CAD build for the part. Positions are in the model's coordinates, mm. Face numbers are marked on the shaded views. A direction names the side the tool comes from. Round coordinates to 2 decimals unless told otherwise and drop trailing zeros. Write each loop counter-clockwise with the first axis right and the second up, starting at its lowest first coordinate (ties: lowest second). Pieces come first, ordered by that corner, then holes. Notation, with made-up numbers: (34.5, -37) - (78.5, -37) arc R17 ccw to (78.5, -4) - close; hole circle Ø5 at (-20.5, -11.75). An arc over 180 degrees is marked (long way). Use one line per item in the form item = value. Start each with the question number.
Item 1: Drill centre lines: L1, parallel to X at y = 18, z = -43.5; L2, parallel to X at y = 23, z = -108; L3, parallel to Z at x = -30.5, y = 20. Where is each one in solid material? Low to high.
Item 2: Band-saw the part on B-B, the plane z = -60. Give the number of separate pieces and of enclosed holes in the cut face, and give its area (4 significant figures).
Item 3: Pull direction X, two halves, no side cores. Call the marked faces 3, 4 and 5: +X half, -X half, draft (parallel to the pull), parting line (faces both ways), or undercut.
Item 4: Pin check, flat tip, straight feed: pin 1 (12 mm diameter, centred on x = 1.5, z = 49, fed in from +Y). Stop position of the tip, or through.
Item 5: Band-saw the part on A-A, the plane x = -16.5. List the corners of the cut face in (y, z).
Item 6: Tool access for the marked faces 1 and 2: list every direction of +Z, -Z, +X, -X, +Y, -Y with a clear straight run to the whole face (end or side of a thin tool).
from build123d import *

# Parameters (mm, degrees)
BOSS_EXTRUDE1_DEPTH     = 6.35
BOSS_EXTRUDE2_DEPTH     = 38.1
CUT_EXTRUDE1_DEPTH      = 12.7
CUT_EXTRUDE1_DEPTH_BACK = 25.4
CUT_EXTRUDE2_DEPTH      = 6.35
CUT_EXTRUDE2_DEPTH_BACK = 25.4
CUT_EXTRUDE3_DEPTH      = 156.552724943
BOSS_EXTRUDE3_DEPTH     = 38.1


with BuildPart() as part:
    # Sketch1 → Boss-Extrude1 (new body)
    with BuildSketch(Plane(origin=(0, 0, 0), x_dir=(1, 0, 0), z_dir=(0, 1, 0))):
        with BuildLine():
            Line((-81.75625, 119.0625), (81.75625, 119.0625))
            ThreePointArc((81.75625, 119.0625), (87.368910076, 116.737660076), (89.69375, 111.125))
            Line((89.69375, 111.125), (89.69375, -93.6625))
            ThreePointArc((89.69375, -93.6625), (82.254262242, -111.623012242), (64.29375, -119.0625))
            Line((64.29375, -119.0625), (-64.29375, -119.0625))
            ThreePointArc((-64.29375, -119.0625), (-82.254262242, -111.623012242), (-89.69375, -93.6625))
            Line((-89.69375, -93.6625), (-89.69375, 111.125))
            ThreePointArc((-89.69375, 111.125), (-87.368910076, 116.737660076), (-81.75625, 119.0625))
        make_face()
    extrude(amount=BOSS_EXTRUDE1_DEPTH)

    # Sketch2 → Boss-Extrude2 (add)
    with BuildSketch(Plane(origin=(0, 6.35, 0), x_dir=(1, 0, 0), z_dir=(0, 1, 0))):
        with BuildLine():
            Line((89.69375, -93.6625), (89.69375, 111.125))
            ThreePointArc((89.69375, 111.125), (87.368910076, 116.737660076), (81.75625, 119.0625))
            Line((81.75625, 119.0625), (-81.75625, 119.0625))
            ThreePointArc((-81.75625, 119.0625), (-87.368910076, 116.737660076), (-89.69375, 111.125))
            Line((-89.69375, 111.125), (-89.69375, -93.6625))
            ThreePointArc((-89.69375, -93.6625), (-82.254262242, -111.623012242), (-64.29375, -119.0625))
            Line((-64.29375, -119.0625), (64.29375, -119.0625))
            ThreePointArc((64.29375, -119.0625), (82.254262242, -111.623012242), (89.69375, -93.6625))
        make_face()
        with BuildLine():
            Line((81.75625, 112.7125), (-81.75625, 112.7125))
            ThreePointArc((-81.75625, 112.7125), (-82.878782015, 112.247532015), (-83.34375, 111.125))
            Line((-83.34375, 111.125), (-83.34375, -93.6625))
            ThreePointArc((-83.34375, -93.6625), (-77.764134182, -107.132884182), (-64.29375, -112.7125))
            Line((-64.29375, -112.7125), (64.29375, -112.7125))
            ThreePointArc((64.29375, -112.7125), (77.764134182, -107.132884182), (83.34375, -93.6625))
            Line((83.34375, -93.6625), (83.34375, 111.125))
            ThreePointArc((83.34375, 111.125), (82.878782015, 112.247532015), (81.75625, 112.7125))
        make_face(mode=Mode.SUBTRACT)
    extrude(amount=BOSS_EXTRUDE2_DEPTH)

    # Sketch5 → Cut-Extrude1 (cut, two sides: drawn at the far end of the back side and taken through both)
    with BuildSketch(Plane(origin=(-13.135345572, 31.711529428, 0), x_dir=(0, 0, 1), z_dir=(-0.38268343236509383, 0.9238795325112852, 0)).offset(-CUT_EXTRUDE1_DEPTH_BACK)):
        with BuildLine():
            Line((-52.21366875, -70.394979916), (-11.28633125, -70.394979916))
            add(Edge.make_bspline(
                [(-11.28633125, -70.394979916), (20.46366875, -70.394979916), (20.46366875, -38.644979916), (-11.28633125, -38.644979916)],
                knots=[0, 0, 0, 0, 1, 1, 1, 1], degree=3, weights=[1, 0.333333333, 0.333333333, 1]))
            Line((-11.28633125, -38.644979916), (-52.21366875, -38.644979916))
            add(Edge.make_bspline(
                [(-52.21366875, -70.394979916), (-83.96366875, -70.394979916), (-83.96366875, -38.644979916), (-52.21366875, -38.644979916)],
                knots=[0, 0, 0, 0, 1, 1, 1, 1], degree=3, weights=[1, 0.333333333, 0.333333333, 1]))
        make_face()
    extrude(amount=CUT_EXTRUDE1_DEPTH + CUT_EXTRUDE1_DEPTH_BACK, mode=Mode.SUBTRACT)

    # Sketch7 → Cut-Extrude2 (cut, two sides: drawn at the far end of the back side and taken through both)
    with BuildSketch(Plane(origin=(13.135345572, 31.711529428, 0), x_dir=(0, 0, -1), z_dir=(0.3826834323650874, 0.9238795325112878, 0)).offset(-CUT_EXTRUDE2_DEPTH_BACK)):
        with BuildLine():
            Line((10.20445, -72.146741698), (53.29555, -72.146741698))
            add(Edge.make_bspline(
                [(53.29555, -40.396741698), (85.04555, -40.396741698), (85.04555, -72.146741698), (53.29555, -72.146741698)],
                knots=[0, 0, 0, 0, 1, 1, 1, 1], degree=3, weights=[1, 0.333333333, 0.333333333, 1]))
            Line((53.29555, -40.396741698), (10.20445, -40.396741698))
            add(Edge.make_bspline(
                [(10.20445, -72.146741698), (-21.54555, -72.146741698), (-21.54555, -40.396741698), (10.20445, -40.396741698)],
                knots=[0, 0, 0, 0, 1, 1, 1, 1], degree=3, weights=[1, 0.333333333, 0.333333333, 1]))
        make_face()
    extrude(amount=CUT_EXTRUDE2_DEPTH + CUT_EXTRUDE2_DEPTH_BACK, mode=Mode.SUBTRACT)

    # Sketch8 → Cut-Extrude3 (cut, through all)
    with BuildSketch(Plane.XZ):
        with BuildLine():
            Line((13.49375, 106.83875), (26.19375, 106.83875))
            ThreePointArc((26.19375, 106.83875), (35.71875, 97.31375), (26.19375, 87.78875))
            Line((26.19375, 87.78875), (13.49375, 87.78875))
            ThreePointArc((13.49375, 87.78875), (3.96875, 97.31375), (13.49375, 106.83875))
        make_face()
        with BuildLine():
            Line((-26.19375, 80.9625), (-13.49375, 80.9625))
            ThreePointArc((-13.49375, 80.9625), (-3.96875, 71.4375), (-13.49375, 61.9125))
            Line((-13.49375, 61.9125), (-26.19375, 61.9125))
            ThreePointArc((-26.19375, 61.9125), (-35.71875, 71.4375), (-26.19375, 80.9625))
        make_face()
    extrude(amount=-CUT_EXTRUDE3_DEPTH, mode=Mode.SUBTRACT)

    # Sketch9 → Boss-Extrude3 (add)
    with BuildSketch(Plane(origin=(0, 6.35, 0), x_dir=(1, 0, 0), z_dir=(0, 1, 0))):
        with BuildLine():
            Line((-81.75625, 112.7125), (-71.120073585, 112.7125))
            ThreePointArc((-71.120073585, 112.7125), (-73.309655038, 111.836708137), (-74.291288385, 109.692489328))
            ThreePointArc((-74.291288385, 109.692489328), (-76.143589924, 105.512339924), (-80.323739328, 103.660038385))
            ThreePointArc((-80.323739328, 103.660038385), (-82.467958137, 102.678405038), (-83.34375, 100.488823585))
            Line((-83.34375, 100.488823585), (-83.34375, 111.125))
            ThreePointArc((-83.34375, 111.125), (-82.878782015, 112.247532015), (-81.75625, 112.7125))
        make_face()
        with BuildLine():
            Line((-9.525, -112.7125), (9.525, -112.7125))
            ThreePointArc((9.525, -112.7125), (7.27993597, -111.78256403), (6.35, -109.5375))
            ThreePointArc((6.35, -109.5375), (0, -103.1875), (-6.35, -109.5375))
            ThreePointArc((-6.35, -109.5375), (-7.27993597, -111.78256403), (-9.525, -112.7125))
        make_face()
        with BuildLine():
            Line((-9.525, 112.7125), (9.525, 112.7125))
            ThreePointArc((9.525, 112.7125), (7.27993597, 111.78256403), (6.35, 109.5375))
            ThreePointArc((6.35, 109.5375), (0, 103.1875), (-6.35, 109.5375))
            ThreePointArc((-6.35, 109.5375), (-7.27993597, 111.78256403), (-9.525, 112.7125))
        make_face()
        with BuildLine():
            Line((83.34375, 111.125), (83.34375, 100.488823585))
            ThreePointArc((83.34375, 100.488823585), (82.467958137, 102.678405038), (80.323739328, 103.660038385))
            ThreePointArc((80.323739328, 103.660038385), (76.143589924, 105.512339924), (74.291288385, 109.692489328))
            ThreePointArc((74.291288385, 109.692489328), (73.309655038, 111.836708137), (71.120073585, 112.7125))
            Line((71.120073585, 112.7125), (81.75625, 112.7125))
            ThreePointArc((81.75625, 112.7125), (82.878782015, 112.247532015), (83.34375, 111.125))
        make_face()
        with BuildLine():
            ThreePointArc((-83.049421546, -96.998258512), (-81.324581361, -99.291426622), (-78.45534091, -99.257472557))
            ThreePointArc((-78.45534091, -99.257472557), (-71.028942091, -100.397692091), (-69.888722557, -107.82409091))
            ThreePointArc((-69.888722557, -107.82409091), (-69.922676622, -110.693331361), (-67.629508512, -112.418171546))
            ThreePointArc((-67.629508512, -112.418171546), (-77.764134182, -107.132884182), (-83.049421546, -96.998258512))
        make_face()
        with BuildLine():
            ThreePointArc((69.888722557, -107.82409091), (69.922676622, -110.693331361), (67.629508512, -112.418171546))
            ThreePointArc((67.629508512, -112.418171546), (77.764134182, -107.132884182), (83.049421546, -96.998258512))
            ThreePointArc((83.049421546, -96.998258512), (81.324581361, -99.291426622), (78.45534091, -99.257472557))
            ThreePointArc((78.45534091, -99.257472557), (71.028942091, -100.397692091), (69.888722557, -107.82409091))
        make_face()
    extrude(amount=BOSS_EXTRUDE3_DEPTH)


solid = part.part
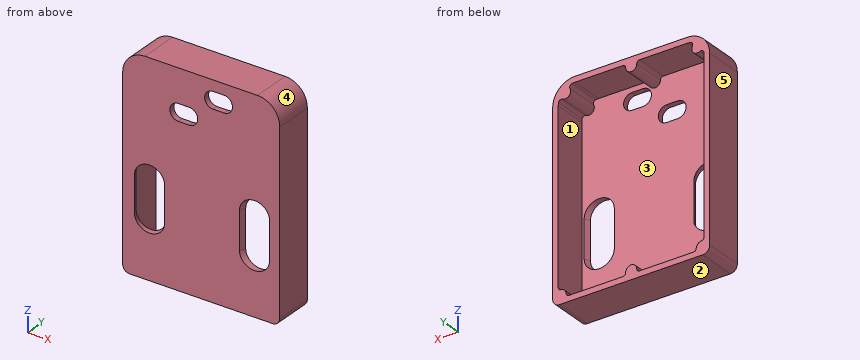
Determined:
q1.L1 = -89.69 to -83.34, 83.34 to 89.69
q1.L2 = -89.69 to -74.61, -6.16 to 6.16, 74.61 to 89.69
q1.L3 = -119.06 to -112.71, 112.71 to 119.06
q2.separate_pieces = 3
q2.enclosed_holes = 0
q2.area = 1,235 mm²
q3.face_3 = undercut
q3.face_4 = +X half
q3.face_5 = -X half
q4.pin_1 = 6.35
q5.outline = (0, -119.06) - (44.45, -119.06) - (44.45, -112.71) - (6.35, -112.71) - (6.35, 61.91) - (0, 61.91) - close; (0, 80.96) - (6.35, 80.96) - (6.35, 112.71) - (44.45, 112.71) - (44.45, 119.06) - (0, 119.06) - close
q6.face_1 = +Y
q6.face_2 = -Z, +X, -X, +Y, -Y
